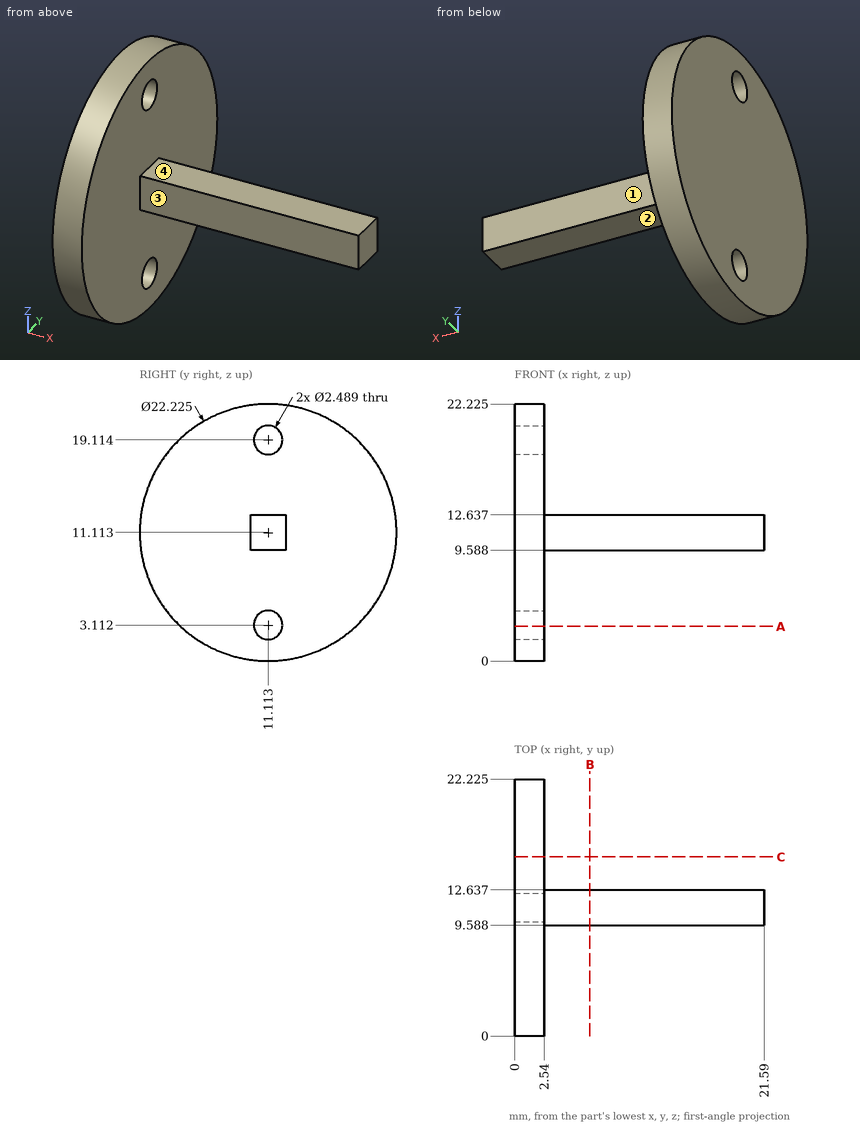
Could you check a few things on this drawing? It's one solid part, dimensions in mm from its lowest x, y, z. A direction names the side the tool comes from. Coordinates: 2 decimals unless noted, no trailing zeros. Write each loop counter-clockwise with the first axis right and the second up, starting at its lowest first coordinate (ties: lowest second). Pieces come first, ordered by that corner, then holes. Notation, with made-up numbers: (58.5, 75) - (93.5, 75) arc R19 cw to (93.5, 86) - close; hole circle Ø11 at (46, -1). An arc over 180 degrees is marked (long way). Return JSON: item names as keys, results as strings. Group by question number.
Item 1: If we section it at A-A (z = 3): Write out the boundary of the cut face in (x, y).
Item 2: I'm going to push flat-ended pins straight in: pin 1 Ø4 at (y, z) = (5, 15) entering from +X; pin 2 Ø10 at (x, y) = (14, 10.5) entering from -Z; pin 3 Ø1.5 at (x, y) = (16, 10.5) entering from +Z. Where does each tip first touch, or does it pass through?
Item 3: If we section it at B-B (x = 6.5): Write out the boundary of the cut face in (y, z).
Item 4: If we section it at C-C (y = 15.5): Write out the boundary of the cut face in (x, z).
Item 5: Please list where these lines run through material, in increasing order: probe 1 along X at (y, z) = (19.5, 9); probe 2 along Z at (x, y) = (12, 10); probe 3 along Y at (x, z) = (1.25, 12.5).
Item 6: Which directions (+Z, -Z, +X, -X, +Y, -Y) give clear straight access to the entire face, cutting with the end or side of a thin tool? Please do the marked faces 1, 2, 3 and 4.
Return value:
{
 "1": {"outline": "(0, 3.52) - (2.54, 3.52) - (2.54, 9.87) - (0, 9.87) - close; (0, 12.35) - (2.54, 12.35) - (2.54, 18.71) - (0, 18.71) - close"},
 "2": {"pin 1": "stops at x = 2.54", "pin 2": "stops at z = 9.59", "pin 3": "stops at z = 12.64"},
 "3": {"outline": "(9.59, 9.59) - (12.64, 9.59) - (12.64, 12.64) - (9.59, 12.64) - close"},
 "4": {"outline": "(0, 0.9) - (2.54, 0.9) - (2.54, 21.32) - (0, 21.32) - close"},
 "5": {"probe 1": "x = 0 to 2.54", "probe 2": "z = 9.59 to 12.64", "probe 3": "y = 0.09 to 22.14"},
 "6": {"face 1": "+Z, -Z, +X, +Y", "face 2": "-Z, +X, +Y, -Y", "face 3": "+Z, -Z, +X, -Y", "face 4": "+Z, +X, +Y, -Y"}
}
